Input: part model. Units: mm. Frame: model coordinates. Face numbers are marked on the shaded views. Round coordinates to 2 decimals unless told otherwise and drop trailing zeros. Loops run counter-clockwise (first coordinate to the right, second up) from the corner with the lowest first, then second, coordinate; pieces in that order, holes last. Notation, with made-up numbers: (1.5, 59) -> (27.5, 59) arc R24 ccw to (27.5, 92) -> close; hole circle Ø8 at (-24.5, -14.75). An arc over 180 degrees is marked (long way). Answer as a JSON object with one key per item and string values.
```python
from build123d import *

# Parameters (mm, degrees)
F0_R        = 3.2004
F0_R_2      = 6.35
F0_R_3      = 5.08
F0_R_4      = 11.2395
F1_DEPTH    = 9.525
F2_W        = 12.7
F2_H        = 5.1071889116
F3_DEPTH    = 9.525
F4_T1_DEPTH = 9.525
F5_R        = 1.27


# Not quite as in the source:
# - a fillet or chamfer that OpenCascade refuses, or shapes differently, is made with other operations: its cross-section is extruded or revolved along the edge and cut away or added


with BuildPart() as f1:
    # F0 (on Top) → F1 (new body)
    with BuildSketch(Plane.XY):
        with BuildLine():
            Line((-5.159375, 19.9821734518), (-40.878125, 10.7596318587))
            ThreePointArc((-40.878125, 10.7596318587), (-49.2125, 0), (-40.878125, -10.7596318587))
            Line((-40.878125, -10.7596318587), (-5.159375, -19.9821734518))
            ThreePointArc((-5.159375, -19.9821734518), (0, -20.6375), (5.159375, -19.9821734518))
            Line((5.159375, -19.9821734518), (40.878125, -10.7596318587))
            ThreePointArc((40.878125, -10.7596318587), (49.2125, 0), (40.878125, 10.7596318587))
            Line((40.878125, 10.7596318587), (5.159375, 19.9821734518))
            ThreePointArc((5.159375, 19.9821734518), (0, 20.6375), (-5.159375, 19.9821734518))
        make_face()
        with Locations((-12.7, -12.7)):
            Circle(F0_R, mode=Mode.SUBTRACT)
        with Locations((12.7, -12.7)):
            Circle(F0_R, mode=Mode.SUBTRACT)
        with Locations((-38.1, 0)):
            Circle(F0_R_2, mode=Mode.SUBTRACT)
        with Locations((-19.05, 0)):
            Circle(F0_R_3, mode=Mode.SUBTRACT)
        with Locations((-12.7, 12.7)):
            Circle(F0_R, mode=Mode.SUBTRACT)
        Circle(F0_R_4, mode=Mode.SUBTRACT)
        with Locations((19.05, 0)):
            Circle(F0_R_3, mode=Mode.SUBTRACT)
        with Locations((38.1, 0)):
            Circle(F0_R_2, mode=Mode.SUBTRACT)
        with Locations((12.7, 12.7)):
            Circle(F0_R, mode=Mode.SUBTRACT)
    extrude(amount=F1_DEPTH)

    # F2 (on face) → F3 (join, through all)
    with BuildSketch(Plane.XY.offset(9.525)):
        with Locations((0, 20.7509055442)):
            Rectangle(F2_W, F2_H)
    extrude(amount=-F3_DEPTH)

    # F4: fillet of radius 12.7 on 2 edges, made by hand

    # F4_s2 → F4_t1 (join)
    with BuildSketch(Plane.XY):
        with BuildLine():
            ThreePointArc((-13.9630832797, 17.7090657484), (-9.6168370541, 19.7724670423), (-6.35, 23.3045))
            Line((-6.35, 23.3045), (-6.35, 19.6747553987))
            Line((-6.35, 19.6747553987), (-13.9630832797, 17.7090657484))
        make_face()
        with BuildLine():
            ThreePointArc((13.9630832797, 17.7090657484), (9.6168370541, 19.7724670423), (6.35, 23.3045))
            Line((6.35, 23.3045), (6.35, 19.6747553987))
            Line((6.35, 19.6747553987), (13.9630832797, 17.7090657484))
        make_face()
    extrude(amount=F4_T1_DEPTH)

    # F5
    f5_edges = [f1.edges().sort_by_distance(p)[0] for p in [
        (-6.35, 23.3045, 4.7625),
        (6.35, 23.3045, 4.7625),
    ]]
    fillet(f5_edges, radius=F5_R)


solid = f1.part
```
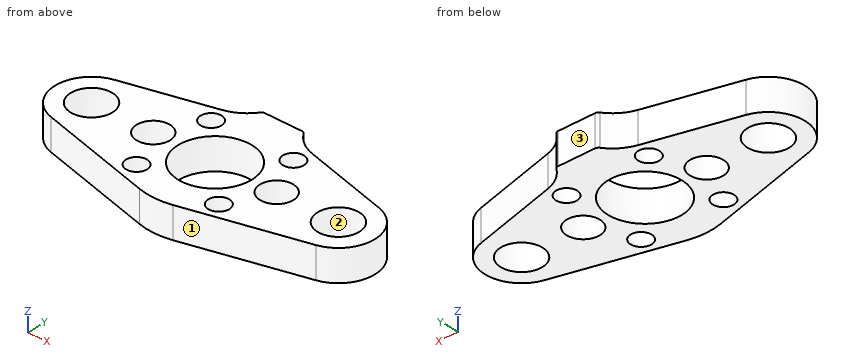
1) Section B-B, the plane x = 0. Output: boundary loops of the cut face in (y, z) (1 decimal), plus the area to 3 significant figures.
Output:
{"outline": "(-20.6, 0) -> (-11.2, 0) -> (-11.2, 9.5) -> (-20.6, 9.5) -> close; (11.2, 0) -> (23.3, 0) -> (23.3, 9.5) -> (11.2, 9.5) -> close", "area": "204 mm^2"}
2) Section D-D, the plane y = -8.5. Output: boundary loops of the cut face in (x, z) (3 decimals), plus the area to 3 significant figures.
Output:
{"outline": "(-45.258, 0) -> (-7.354, 0) -> (-7.354, 9.525) -> (-45.258, 9.525) -> close; (7.354, 0) -> (45.258, 0) -> (45.258, 9.525) -> (7.354, 9.525) -> close", "area": "722 mm^2"}
3) Contact query for flat-ended pins moving along their axis: P1, Ø11.5, axis at x = -38.1, y = 0, coming from the -Z side; P2, Ø1.5, axis at x = -31, z = 8.5, coming from the -Y side; P3, Ø1.5, axis at y = 10.5, z = 4.5, coming from the +X side; P4, Ø4, axis at x = -12, z = 8, coming from the -Y side. Output: stop coordinate, or through.
Output:
{"P1": "passes through", "P2": "stops at y = -13.5", "P3": "stops at x = 43.43", "P4": "stops at y = -18.73"}
4) Section A-A, the plane y = 0. Count the separate pieces of the cut face and the enclosed holes in it, plus the area to 3 significant figures.
Output:
{"separate pieces": "6", "enclosed holes": "0", "area": "288 mm^2"}
5) Ray query, probe 1 along X at (y, z) = (3, 4.75); probe 2 along X at (y, z) = (1, 4); probe 3 along Y at (x, z) = (-12.7, 4.5). Return the intervals inside material, ascending.
Output:
{"probe 1": "x = -48.8 to -43.7, -32.5 to -23.15, -14.95 to -10.83, 10.83 to 14.95, 23.15 to 32.5, 43.7 to 48.8", "probe 2": "x = -49.17 to -44.37, -31.83 to -24.03, -14.07 to -11.19, 11.19 to 14.07, 24.03 to 31.83, 44.37 to 49.17", "probe 3": "y = -18.04 to -15.9, -9.5 to 9.5, 15.9 to 18.11"}
6) Draft query along X for the marked faces 1, 2 and 3. Return one class per face: +X half, -X half, draft (parallel to the pull), parting line (faces both ways), or undercut.
Output:
{"face 1": "+X half", "face 2": "undercut", "face 3": "draft"}
